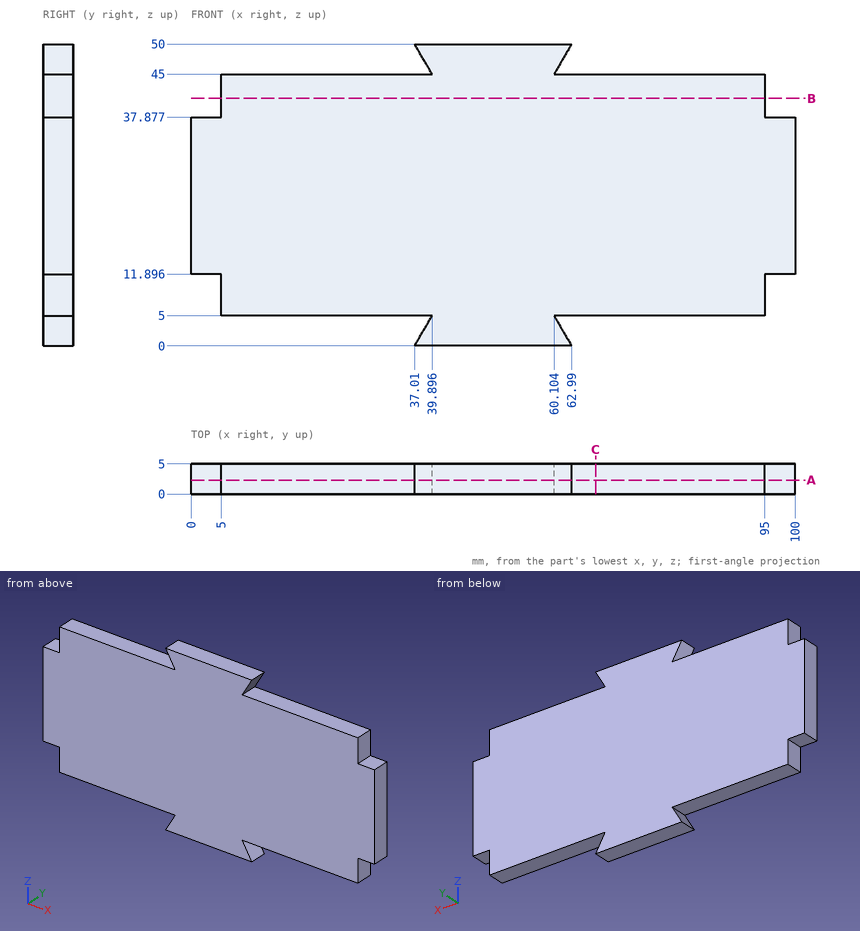
Source: three-view drawing plus pictorial views. Frame: mm from the lowest corner of the part. Round coordinates to 2 decimals unless told otherwise and drop trailing zeros. Loops run counter-clockwise (first coordinate to the right, second up) from the corner with the lowest first, then second, coordinate; pieces in that order, holes last. Notation, with made-up numbers: (-19, 80) - (10, 80) arc R32 ccw to (10, 117) - close; hole circle Ø1 at (-12, 12). An arc over 180 degrees is marked (long way). Write each question's results on one line, items separated by ' | '. Start each with the question number.
1) First-contact query: P1, Ø2.5, axis at x = 85, y = 1.5, coming from the -Z side; P2, Ø1.5, axis at x = 98, y = 3, coming from the -Z side; P3, Ø1.5, axis at y = 2.5, z = 42, coming from the +X side. Flat tips, straight axial feed; report the tip coordinate or a pass-through.
2) Line query: probe 1 along Z at (x, y) = (35, 3.3); probe 2 along X at (y, z) = (4.3, 44.5); probe 3 along X at (y, z) = (3, 4). Output: solid intervals per line, ascending. Write a range as [from, to].
3) Cut plane A-A on y = 2.3. Return loops of the section in (x, z), then the cut area to 3 significant figures.
4) Cut plane C-C on x = 67. Return loops of the section in (y, z).
5) Cut plane B-B on z = 41. Return loops of the section in (x, y), then the cut area to 3 significant figures.
Verdict:
1) P1: stops at z = 5 | P2: stops at z = 11.9 | P3: stops at x = 95
2) probe 1: z = [5, 45] | probe 2: x = [5, 95] | probe 3: x = [39.32, 60.68]
3) outline: (0, 11.9) - (5, 11.9) - (5, 5) - (39.9, 5) - (37.01, 0) - (62.99, 0) - (60.1, 5) - (95, 5) - (95, 11.9) - (100, 11.9) - (100, 37.88) - (95, 37.88) - (95, 45) - (60.1, 45) - (62.99, 50) - (37.01, 50) - (39.9, 45) - (5, 45) - (5, 37.88) - (0, 37.88) - close | area: 4,090 mm2
4) outline: (0, 5) - (5, 5) - (5, 45) - (0, 45) - close
5) outline: (5, 0) - (95, 0) - (95, 5) - (5, 5) - close | area: 450 mm2
